Job drawing, mm, ordinate dimensions from the low corner. One solid piece. A direction names the side the tool comes from. Round coordinates to 2 decimals unless told otherwise and drop trailing zeros. Loops run counter-clockwise (first coordinate to the right, second up) from the corner with the lowest first, then second, coordinate; pieces in that order, holes last. Notation, with made-up numbers: M 73.25,-29 L 102.25,-29 A7 cw 102.25,-23 Z; hole C 31,36.5 d3. An arc over 180 degrees is marked long. Use one line per item in the form item = value. Start each with the question number.
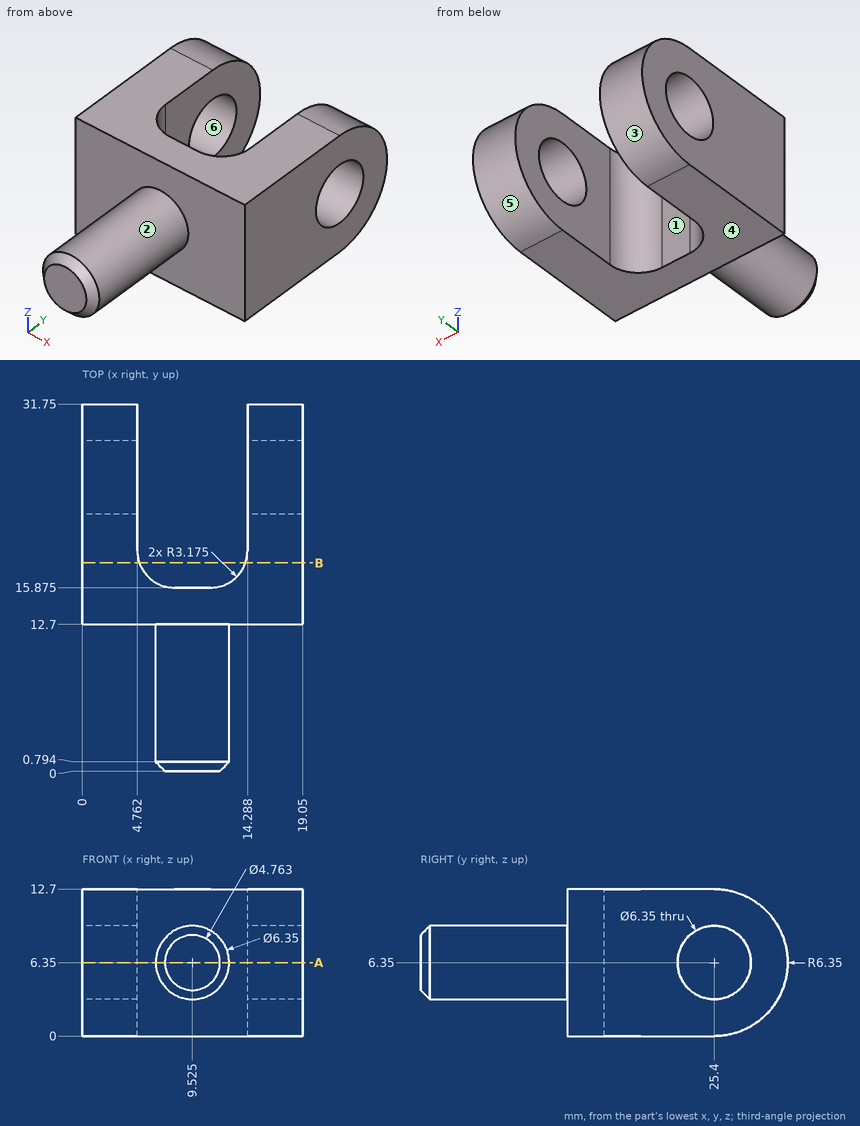
Q1. Saw through at A-A (z = 6.35). Give the number of separate pieces and of enclosed holes in the cut face.
Q2. Saw through at B-B (y = 18). Give the cut face in (x, z).
Q3. Tool access for the marked faces 1, 2 and 3: list every direction of +Z, -Z, +X, -X, +Y, -Y with a clear straight run to the whole face (end or side of a thin tool).
Q4. Drop a flat-ended pin along its axis: P1, Ø2.5, axis at x = 9.5, z = 9, coming from the +Y side (1 decimal). Give the stop position or say it passes through.
Q5. Wall check: probe 1 along X at (y, z) = (19, 9.25); probe 2 along Z at (x, y) = (16.2, 25.4) (1 decimal); probe 3 along X at (y, z) = (18, 9.75). Give the ranges that are in metal, low to high.
Q6. Pull direction Z, two halves, no side cores. Call the marked faces 4, 5 and 6: pulls with the +Z half, pulls with the -Z half, needs draft (parallel to the pull), parting line crosses it, or undercut.
Filled in:
q1.separate_pieces = 3
q1.enclosed_holes = 0
q2.outline = M 0,0 L 4.94,0 L 4.94,12.7 L 0,12.7 Z; M 14.11,0 L 19.05,0 L 19.05,12.7 L 14.11,12.7 Z
q3.face_1 = +Z, -Z, +Y
q3.face_2 = -Y
q3.face_3 = +X, -X, +Y
q4.P1 = 15.9
q5.probe_1 = 0 to 4.76, 14.29 to 19.05
q5.probe_2 = 0 to 3.2, 9.5 to 12.7
q5.probe_3 = 0 to 4.94, 14.11 to 19.05
q6.face_4 = pulls with the -Z half
q6.face_5 = parting line crosses it
q6.face_6 = undercut
